Source: CAD feature listing. Evaluate the final solid. Frame: model axes, mm. A direction names the side the tool comes from. Coordinates: 2 decimals unless noted, no trailing zeros. Loops run counter-clockwise (first coordinate to the right, second up) from the corner with the lowest first, then second, coordinate; pieces in that order, holes last. Notation, with made-up numbers: (-18, -15) -> (18, -15) arc R9 ccw to (18, -2) -> close; hole circle Ø3 at (34.25, -23.5). An arc over 180 degrees is marked (long way). Answer as CSV lines item,"result".
from build123d import *

# Parameters (mm, degrees)
SKETCH1_R           = 7.5
BOSS_EXTRUDE1_DEPTH = 70
SKETCH2_R           = 10.194447781
SKETCH2_R_2         = 5
CUT_EXTRUDE1_DEPTH  = 19
CUT_EXTRUDE2_START  = -19
SKETCH3_R           = 9.951910859
SKETCH3_R_2         = 5
CUT_EXTRUDE2_DEPTH  = 19
SKETCH4_R           = 2.5
CUT_EXTRUDE3_DEPTH  = 10
CUT_EXTRUDE4_START  = -10
SKETCH5_R           = 2.5
CUT_EXTRUDE4_DEPTH  = 10


with BuildPart() as part:
    # Sketch1 → Boss-Extrude1 (new body)
    with BuildSketch(Plane.XY):
        Circle(SKETCH1_R)
    extrude(amount=BOSS_EXTRUDE1_DEPTH)

    # Sketch2 → Cut-Extrude1 (cut)
    with BuildSketch(Plane(origin=(0, 0, 0), x_dir=(-1, 0, 0), z_dir=(0, 0, -1))):
        Circle(SKETCH2_R)
        Circle(SKETCH2_R_2, mode=Mode.SUBTRACT)
    extrude(amount=-CUT_EXTRUDE1_DEPTH, mode=Mode.SUBTRACT)

    # Sketch3 → Cut-Extrude2 (cut)
    with BuildSketch(Plane.XY.offset(70).offset(CUT_EXTRUDE2_START)):
        Circle(SKETCH3_R)
        with Locations(Location((0, 0, 0), (0, 0, 180))):
            Circle(SKETCH3_R_2, mode=Mode.SUBTRACT)
    extrude(amount=CUT_EXTRUDE2_DEPTH, mode=Mode.SUBTRACT)

    # Sketch4 → Cut-Extrude3 (cut)
    with BuildSketch(Plane.XY.offset(70)):
        Circle(SKETCH4_R)
    extrude(amount=-CUT_EXTRUDE3_DEPTH, mode=Mode.SUBTRACT)

    # Sketch5 → Cut-Extrude4 (cut)
    with BuildSketch(Plane(origin=(0, 0, 0), x_dir=(-1, 0, 0), z_dir=(0, 0, -1)).offset(CUT_EXTRUDE4_START)):
        with Locations(Location((0, 0, 0), (0, 0, 180))):
            Circle(SKETCH5_R)
    extrude(amount=CUT_EXTRUDE4_DEPTH, mode=Mode.SUBTRACT)


solid = part.part
(1) Access query for faces 1 (the cylindrical face through (-7.493, 0.33, 34.776)), 2 (the cylindrical face through (-0.54, -2.44, 65.07)), 3 (the cylindrical face through (1.08, -4.88, 9.37)). Directions: +Z, -Z, +X, -X, +Y, -Y. A direction counts if a zero-diameter tool reaches every point of the face in a straight line with its end or side. Return the directions, or none.
Computed values:
face 1,"+Z, -Z"
face 2,"+Z"
face 3,"-Z"
(2) Pin query (flat end, axial travel): pin 1 Ø8 at (x, z) = (-3, 13.5) entering from +Y; pin 2 Ø6 at (x, z) = (1, 58) entering from -Y; pin 3 Ø1.5 at (x, y) = (1, 0) entering from +Z. Return the tip coordinate at first contact, or that it passes through.
Computed values:
pin 1,"y = 5"
pin 2,"y = -5"
pin 3,"z = 60"
(3) Cut plane D-D (z = 34). Return the cut outline in (x, y).
Computed values:
outline,"circle Ø15 at (0, 0)"
(4) Cut plane A-A (x = 0). Return the cut outline in (y, z).
Computed values:
outline,"(-7.5, 19) -> (-5, 19) -> (-5, 0) -> (-2.5, 0) -> (-2.5, 10) -> (2.5, 10) -> (2.5, 0) -> (5, 0) -> (5, 19) -> (7.5, 19) -> (7.5, 51) -> (5, 51) -> (5, 70) -> (2.5, 70) -> (2.5, 60) -> (-2.5, 60) -> (-2.5, 70) -> (-5, 70) -> (-5, 51) -> (-7.5, 51) -> close"
(5) Cut plane C-C (z = 63.5). Return the cut outline in (x, y).
Computed values:
outline,"circle Ø10 at (0, 0); hole circle Ø5 at (0, 0)"
(6) Material intervals for L1, parallel to Y at x = 0, z = 2.5; L2, parallel to Z at x = 5.75, y = -4.5; L3, parallel to Y at x = -0.25, z = 58, sorted ascending. Write a range as [from, to].
Computed values:
L1,"[-5, -2.5], [2.5, 5]"
L2,"[19, 51]"
L3,"[-4.99, 4.99]"
(7) Draft query along X for faces 4 (the cylindrical face through (5, 0, 60)), 5 (the cylindrical face through (-2.5, -0.1, 5.1)), 6 (the flat face through (2, -2, 70)). Return one class per face: released by +X, released by -X, zero draft, split by the parting line, or undercut.
Computed values:
face 4,"split by the parting line"
face 5,"undercut"
face 6,"zero draft"
